from build123d import *

# Parameters (mm, degrees)
BOSS_EXTRUDE1_DEPTH = 1500
SKETCH5_R           = 52.5
CUT_EXTRUDE3_DEPTH  = 30
LPATTERN2_COUNT     = 4
LPATTERN2_PITCH     = 366
SKETCH6_R           = 7
CUT_EXTRUDE4_DEPTH  = 1515.807183702
LPATTERN3_COUNT     = 4
LPATTERN3_PITCH     = 366


with BuildPart() as part:
    # Sketch1 → Boss-Extrude1 (new body)
    with BuildSketch(Plane(origin=(0, 0, 0), x_dir=(0, 0, -1), z_dir=(1, 0, 0))):
        with BuildLine():
            Line((-86.622073579, 113.879598662), (-186.622073579, 113.879598662))
            Line((-186.622073579, 113.879598662), (-186.622073579, -186.120401338))
            Line((-186.622073579, -186.120401338), (-86.622073579, -186.120401338))
            Line((-86.622073579, -186.120401338), (-86.622073579, -180.120401338))
            ThreePointArc((-86.622073579, -180.120401338), (-89.551005767, -173.049333526), (-96.622073579, -170.120401338))
            Line((-96.622073579, -170.120401338), (-166.622073579, -170.120401338))
            ThreePointArc((-166.622073579, -170.120401338), (-173.69314139, -167.19146915), (-176.622073579, -160.120401338))
            Line((-176.622073579, -160.120401338), (-176.622073579, 87.879598662))
            ThreePointArc((-176.622073579, 87.879598662), (-173.69314139, 94.950666474), (-166.622073579, 97.879598662))
            Line((-166.622073579, 97.879598662), (-96.622073579, 97.879598662))
            ThreePointArc((-96.622073579, 97.879598662), (-89.551005767, 100.80853085), (-86.622073579, 107.879598662))
            Line((-86.622073579, 107.879598662), (-86.622073579, 113.879598662))
        make_face()
    extrude(amount=BOSS_EXTRUDE1_DEPTH)

    # Sketch5 → Cut-Extrude3 (cut)
    with BuildSketch(Plane(origin=(0, 0, 176.622073579), x_dir=(-1, 0, 0), z_dir=(0, 0, -1))):
        with Locations(Location((-1299, -36.120401338, 0), (0, 0, 90))):
            Circle(SKETCH5_R)
    cut_extrude3 = extrude(amount=-CUT_EXTRUDE3_DEPTH, mode=Mode.SUBTRACT)

    # LPattern2: Cut-Extrude3 ×4
    with Locations(*[(-i * LPATTERN2_PITCH, 0, 0) for i in range(1, LPATTERN2_COUNT)]):
        add(cut_extrude3, mode=Mode.SUBTRACT)

    # Sketch6 → Cut-Extrude4 (cut, symmetric)
    with BuildSketch(Plane.XY.offset(186.622073579)):
        with Locations(Location((1347.436814511, 12.316413173, 0), (0, 0, 270))):
            Circle(SKETCH6_R)
        with Locations(Location((1347.436814511, -84.557215849, 0), (0, 0, 270))):
            Circle(SKETCH6_R)
    cut_extrude4 = extrude(amount=CUT_EXTRUDE4_DEPTH, both=True, mode=Mode.SUBTRACT)

    # LPattern3: Cut-Extrude4 ×4
    with Locations(*[(-i * LPATTERN3_PITCH, 0, 0) for i in range(1, LPATTERN3_COUNT)]):
        add(cut_extrude4, mode=Mode.SUBTRACT)


solid = part.part
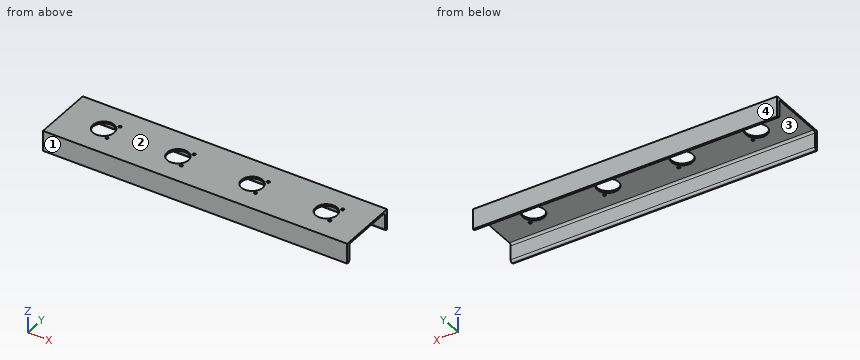
Could you check a few things on this model? Use its own coordinates, in mm. Face numbers are marked on the shaded views. Give positions to 0.01 mm unless a question says otherwise; leave off trailing zeros. Order: outer loops, then holes, each group sorted by start corner. A loop starts at its lowest first (then second) coordinate and runs counter-clockwise, first axis right, second up.
1. Suppose I cut it at D-D (x = 224). Write out the boundary of the cut face in (y, z), plus the area to 3 significant figures.
Answers below:
outline: (-186.12, 86.62) - (-180.12, 86.62) arc R10 ccw to (-170.12, 96.62) - (-170.12, 166.62) arc R10 cw to (-160.12, 176.62) - (-83.31, 176.62) - (-83.31, 186.62) - (-186.12, 186.62) - close; (11.07, 176.62) - (87.88, 176.62) arc R10 cw to (97.88, 166.62) - (97.88, 96.62) arc R10 ccw to (107.88, 86.62) - (113.88, 86.62) - (113.88, 186.62) - (11.07, 186.62) - close
area: 4,940 mm2
2. Suppose I cut it at A-A (z = 126.5). Write out the boundary of the cut face in (x, y), plus the area to 3 significant figures.
Answers below:
outline: (0, -186.12) - (1500, -186.12) - (1500, -170.12) - (0, -170.12) - close; (0, 97.88) - (1500, 97.88) - (1500, 113.88) - (0, 113.88) - close
area: 48,000 mm2
3. Suppose I cut it at C-C (x = 1059). Write out the boundary of the cut face in (y, z).
Answers below:
outline: (-186.12, 86.62) - (-180.12, 86.62) arc R10 ccw to (-170.12, 96.62) - (-170.12, 166.62) arc R10 cw to (-160.12, 176.62) - (87.88, 176.62) arc R10 cw to (97.88, 166.62) - (97.88, 96.62) arc R10 ccw to (107.88, 86.62) - (113.88, 86.62) - (113.88, 186.62) - (-186.12, 186.62) - close
4. I need wall thicknesses on L1, parallel to Y at x = 496, z = 117; L2, parallel to Z at x = 1118, y = -49.5; L3, parallel to Y at x = 202, z = 94. Which ranges of each line are inside material? Lowest first, please.
Answers below:
L1: y = -186.12 to -170.12, 97.88 to 113.88
L2: z = 176.62 to 186.62
L3: y = -186.12 to -170.47, 98.23 to 113.88
5. Suppose I cut it at B-B (x = 567). Write out the boundary of the cut face in (y, z), plus the area to 3 significant figures.
Answers below:
outline: (-186.12, 86.62) - (-180.12, 86.62) arc R10 ccw to (-170.12, 96.62) - (-170.12, 166.62) arc R10 cw to (-160.12, 176.62) - (-88.62, 176.62) - (-88.62, 186.62) - (-186.12, 186.62) - close; (16.38, 176.62) - (87.88, 176.62) arc R10 cw to (97.88, 166.62) - (97.88, 96.62) arc R10 ccw to (107.88, 86.62) - (113.88, 86.62) - (113.88, 186.62) - (16.38, 186.62) - close
area: 4,830 mm2
6. Thinking about a two-plate mould opening in Y: for the marked faces 1, 2, 3 and 4, which applies, +Y half, -Y half, draft (parallel to the pull), parting line (faces both ways), or undercut?
Answers below:
face 1: -Y half
face 2: draft
face 3: undercut
face 4: +Y half
7. For pin 1 (16 mm diameter, centred on x = 1347.44, y = 12.32, fed in from +Z); pin 2 (22.5 mm diameter, centred on x = 615.44, y = 12.32, fed in from -Z), each with a flat end and sliding along its axis, tell me the tip position at first contact or that it passes through.
Answers below:
pin 1: stops at z = 186.62
pin 2: stops at z = 176.62
